```python
from build123d import *

# Parameters (mm, degrees)
F0_R     = 1.5875
F1_DEPTH = 3.175


with BuildPart() as f1:
    # F0 (on Top) → F1 (new body)
    with BuildSketch(Plane.XY):
        with BuildLine():
            Line((19.05, 0), (6.35, 0))
            ThreePointArc((6.35, 0), (1.859872, -1.859872), (0, -6.35))
            Line((0, -6.35), (0, -38.1))
            Line((0, -38.1), (25.4, -38.1))
            Line((25.4, -38.1), (25.4, -6.35))
            ThreePointArc((25.4, -6.35), (23.540128, -1.859872), (19.05, 0))
        make_face()
        with Locations((12.7, -12.7)):
            Circle(F0_R, mode=Mode.SUBTRACT)
    extrude(amount=F1_DEPTH)


solid = f1.part
```
Geometry: final body of the model. Coordinates: model frame, mm. Give positions to 0.01 mm unless a question says otherwise; leave off trailing zeros. Order: outer loops, then holes, each group sorted by start corner. A loop starts at its lowest first (then second) coordinate and runs counter-clockwise, first axis right, second up. Notation, with made-up numbers: (5, 11) -> (45, 11) arc R22 ccw to (45, 36) -> close; hole circle Ø6 at (60, 12). An arc over 180 degrees is marked (long way). Write each question's results on one line, items separated by ' | '. Start each with the question number.
1) Line query: line 1 (Y direction, x = 12.7, z = 0.9); line 2 (X direction, y = -13.5, z = 0.95); line 3 (Y direction, x = 11.5, z = 1.25). Output: solid intervals per line, ascending. Write a range as from..to.
2) Section D-D (x = 3). Return loops of the section in (y, z) (3 decimals).
3) Section B-B (x = 12.7). Return loops of the section in (y, z) (1 decimal).
4) Draft query along Y for faces 1 (the cylindrical face through (14.214, -12.223, 1.565)), 2 (the flat face through (13, -38.1, 2)), 3 (the flat face through (25.4, -22, 2)). Return one class per face: pulls with the +Y half, pulls with the -Y half, needs draft (parallel to the pull), parting line crosses it, or undercut.
5) Section A-A (y = -12.7). Return loops of the section in (x, z) (1 decimal).
Calculated:
1) line 1: -38.1..-14.29, -11.11..0 | line 2: 0..11.33, 14.07..25.4 | line 3: -38.1..-13.74, -11.66..0
2) outline: (-38.1, 0) -> (-0.956, 0) -> (-0.956, 3.175) -> (-38.1, 3.175) -> close
3) outline: (-38.1, 0) -> (-14.3, 0) -> (-14.3, 3.2) -> (-38.1, 3.2) -> close; (-11.1, 0) -> (0, 0) -> (0, 3.2) -> (-11.1, 3.2) -> close
4) face 1: undercut | face 2: pulls with the -Y half | face 3: needs draft
5) outline: (0, 0) -> (11.1, 0) -> (11.1, 3.2) -> (0, 3.2) -> close; (14.3, 0) -> (25.4, 0) -> (25.4, 3.2) -> (14.3, 3.2) -> close
